```python
from build123d import *

# Parameters (mm, degrees)
F1_DEPTH  = 20
F3_DEPTH  = 20
F4_W      = 20
F4_H      = 20
F5_DEPTH  = 20
F6_W      = 20
F6_H      = 20
F7_DEPTH  = 20
F8_W      = 260
F8_H      = 10
F9_DEPTH  = 10
F10_W     = 300
F10_H     = 10
F10_W_2   = 280
F11_DEPTH = 10


with BuildPart() as f1:
    # F0 (on Right) → F1 (new body)
    with BuildSketch(Plane.YZ):
        Polygon((-150, -250), (150, -250), (150, 250), (-50, 250), (-50, -130), (-150, -130), align=None)
    extrude(amount=F1_DEPTH)

    # F2 (on face) → F3 (join)
    with BuildSketch(Plane.YZ.offset(20)):
        with BuildLine():
            Line((-50, 120), (-50, 250))
            Line((-50, 250), (-150, 250))
            Line((-150, 250), (-150, 150))
            Line((-150, 150), (-130, 150))
            ThreePointArc((-130, 150), (-87.279981, 142.253383), (-50, 120))
        make_face()
    extrude(amount=-F3_DEPTH)

    # F4 (on face) → F5 (cut, through all)
    with BuildSketch(Plane.YZ.offset(20)):
        with Locations((140, -200)):
            Rectangle(F4_W, F4_H)
        with Locations((140, -160)):
            Rectangle(F4_W, F4_H)
        with Locations((140, -120)):
            Rectangle(F4_W, F4_H)
        with Locations((140, -80)):
            Rectangle(F4_W, F4_H)
        with Locations((140, -40)):
            Rectangle(F4_W, F4_H)
        with Locations((140, 0)):
            Rectangle(F4_W, F4_H)
        with Locations((140, 40)):
            Rectangle(F4_W, F4_H)
        with Locations((140, 80)):
            Rectangle(F4_W, F4_H)
        with Locations((140, 120)):
            Rectangle(F4_W, F4_H)
        with Locations((140, 160)):
            Rectangle(F4_W, F4_H)
        with Locations((140, 200)):
            Rectangle(F4_W, F4_H)
        with Locations((140, 240)):
            Rectangle(F4_W, F4_H)
        with Locations((140, -240)):
            Rectangle(F4_W, F4_H)
    extrude(amount=-F5_DEPTH, mode=Mode.SUBTRACT)

    # F6 (on face) → F7 (cut, through all)
    with BuildSketch(Plane.YZ.offset(20)):
        with Locations((-140, -200)):
            Rectangle(F6_W, F6_H)
        with Locations((-140, -160)):
            Rectangle(F6_W, F6_H)
        with Locations((-140, -240)):
            Rectangle(F6_W, F6_H)
    extrude(amount=-F7_DEPTH, mode=Mode.SUBTRACT)

    # F8 (on face) → F9 (cut)
    with BuildSketch(Plane(origin=(0, 0, 0), x_dir=(0, -1, 0), z_dir=(-1, 0, 0))):
        with Locations((0, -235)):
            Rectangle(F8_W, F8_H)
    extrude(amount=-F9_DEPTH, mode=Mode.SUBTRACT)

    # F10 (on face) → F11 (cut)
    with BuildSketch(Plane(origin=(0, 0, 0), x_dir=(0, -1, 0), z_dir=(-1, 0, 0))):
        with Locations((0, 245)):
            Rectangle(F10_W, F10_H)
        with Locations((0, 155)):
            Rectangle(F10_W, F10_H)
        with Locations((0, 85)):
            Rectangle(F10_W_2, F10_H)
        with Locations((0, 15)):
            Rectangle(F10_W_2, F10_H)
    extrude(amount=-F11_DEPTH, mode=Mode.SUBTRACT)


solid = f1.part
```
Could you check a few things on this model? Use its own coordinates, in mm. A direction names the side the tool comes from. Give positions to 0.01 mm unless a question says otherwise; leave off trailing zeros. Order: outer loops, then holes, each group sorted by start corner. A loop starts at its lowest first (then second) coordinate and runs counter-clockwise, first axis right, second up.
Q1. If I drill on line 1 along Z through (x, y) = (13.75, -132); line 2 along Z through (x, y) = (9.25, 45); line 3 along Z through (x, y) = (8, -92.5), over which ranges is the centre line in solid material (lowest first)?
Q2. Suppose I cut it at C-C, the plane y = 23. Write out the boundary of the cut face in (x, z).
Q3. For faces 1 (the flat face through (10, 130, 0)), 2 (the flat face through (5, 46, 20)), 3 (the flat face through (5, 41, 80)), 4 (the flat face through (12, -130, -242)), 5 (the flat face through (10, -140, -170)), which set-ups out of +Z, -Z, +X, -X, +Y, -Y let a thin tool reach every point of the face, with its end or its side?
Q4. We'd pull the mould along Z, two halves only. Please class faces 6 (the flat face through (10, 150, 60)), 7 (the flat face through (10, -140, -150)): +Z half, -Z half, draft (parallel to the pull), parting line (faces both ways), or undercut.
Q5. I'm going to push flat-ended pins straight in: P1, Ø6, axis at x = 10.5, y = 141, coming from the -Z side; P2, Ø10, axis at x = 10, z = -201.5, coming from the -Y side; P3, Ø4, axis at x = 2, z = 97.5, coming from the -Y side. Where does each tip first touch, or does it pass through?
Q6. Suppose I cut it at B-B, the plane x = 4.75. Count the separate pieces of the cut face and the enclosed holes in it, and give its area (3 significant figures).
Q7. Suppose I cut it at D-D, the plane z = -57.5. Write out the boundary of the cut face in (x, y).
Q8. Suppose I cut it at A-A, the plane y = -118. Write out the boundary of the cut face in (x, z).
Solution:
1. line 1: z = -230 to -210, -190 to -170, -150 to -130, 150 to 250
1. line 2: z = -250 to -240, -230 to 10, 20 to 80, 90 to 150, 160 to 240
1. line 3: z = -250 to -240, -230 to -130, 144.08 to 150, 160 to 240
2. outline: (0, -250) - (20, -250) - (20, 250) - (10, 250) - (10, 240) - (0, 240) - (0, 160) - (10, 160) - (10, 150) - (0, 150) - (0, 90) - (10, 90) - (10, 80) - (0, 80) - (0, 20) - (10, 20) - (10, 10) - (0, 10) - (0, -230) - (10, -230) - (10, -240) - (0, -240) - close
3. face 1: +X, -X, +Y
3. face 2: -X, -Y
3. face 3: -X, +Y, -Y
3. face 4: -Z, +X, -X, -Y
3. face 5: +X, -X, -Y
4. face 6: draft
4. face 7: undercut
5. P1: stops at z = -230
5. P2: stops at y = -130
5. P3: stops at y = -50
6. separate pieces: 5
6. enclosed holes: 0
6. area: 104,000 mm2
7. outline: (0, -50) - (20, -50) - (20, 150) - (0, 150) - close
8. outline: (0, -250) - (20, -250) - (20, -130) - (0, -130) - (0, -230) - (10, -230) - (10, -240) - (0, -240) - close; (0, 149.41) - (20, 149.41) - (20, 250) - (10, 250) - (10, 240) - (0, 240) - (0, 160) - (10, 160) - (10, 150) - (0, 150) - close
